Build history of the part. All positions in model axes, mm. A direction names the side the tool comes from. Give positions to 0.01 mm unless a question says otherwise; leave off trailing zeros. Order: outer loops, then holes, each group sorted by start corner. A loop starts at its lowest first (then second) coordinate and runs counter-clockwise, first axis right, second up. Notation, with made-up numbers: (53, 10) - (67, 10) arc R28 cw to (67, 49) - close; hole circle Ø5 at (68, -19). An arc over 180 degrees is marked (long way). Answer in a Markdown table with one row per item.
```python
from build123d import *

# Parameters (mm, degrees)
EXTRUDE_1_DEPTH = 100
SKETCH_2_R      = 10
EXTRUDE_2_DEPTH = 100
FILLET_1_R      = 5


with BuildPart() as part:
    # 草图1 → 凸台-拉伸1 (new body)
    with BuildSketch(Plane(origin=(0, 0, 0), x_dir=(1, 0, 0), z_dir=(0, 1, 0))):
        with BuildLine():
            Line((0, 0), (150, 0))
            Line((150, 0), (150, -400))
            ThreePointArc((150, -400), (75, -475), (0, -400))
            Line((0, -400), (0, 0))
        make_face()
    extrude(amount=EXTRUDE_1_DEPTH)

    # 草图2 → 凸台-拉伸2 (add)
    with BuildSketch(Plane(origin=(0, 100, 0), x_dir=(1, 0, 0), z_dir=(0, 1, 0))):
        with Locations((75, -400)):
            Circle(SKETCH_2_R)
    extrude(amount=EXTRUDE_2_DEPTH)

    # 圆角1
    fillet_1_edges = [part.edges().sort_by_distance(p)[0] for p in [
        (65, 200, 400),
    ]]
    fillet(fillet_1_edges, radius=FILLET_1_R)


solid = part.part
```
1. Cut at B-B on y = 67. Write the cut outline in (x, z), and give its area (3 significant figures).
Check result:
| item | result |
|---|---|
| outline | (0, 0) - (150, 0) - (150, 400) arc R75 ccw to (0, 400) - close |
| area | 68,800 mm² |
2. Cut at A-A on z = 197.5. Write the cut outline in (x, y).
Check result:
| item | result |
|---|---|
| outline | (0, 0) - (150, 0) - (150, 100) - (0, 100) - close |
3. Probe line 1 (Y direction, x = 106, z = 56); line 2 (Z direction, x = 34.5, y = 35.5); line 3 (Z direction, x = 99, y = 76.5). List the from-to ranges inside material, lowest first.
Check result:
| item | result |
|---|---|
| line 1 | y = 0 to 100 |
| line 2 | z = 0 to 463.12 |
| line 3 | z = 0 to 471.06 |
4. Cut at C-C on y = 148.5. Write the cut outline in (x, z).
Check result:
| item | result |
|---|---|
| outline | circle Ø20 at (75, 400) |
5. Drop a flat-ended pin along its axis: P1, Ø6, axis at x = 96.5, z = 344, coming from the +Y side. Give the stop position or say it passes through.
Check result:
| item | result |
|---|---|
| P1 | stops at y = 100 |
6. Which spindle directions (+Z, -Z, +X, -X, +Y, -Y) get a long thin tool onto all of the face, cutting with end or side? Do faces 1 (the face through (150, 49, 197)), 2 (the face through (73.698, 146.835, 390.085)). Say none if no direction does.
Check result:
| item | result |
|---|---|
| face 1 | +Z, -Z, +X, +Y, -Y |
| face 2 | +Y |
